Could you check a few things on this model? Use its own coordinates, in mm. A direction names the side the tool comes from. Coordinates: 2 decimals unless noted, no trailing zeros. Loops run counter-clockwise (first coordinate to the right, second up) from the corner with the lowest first, then second, coordinate; pieces in that order, holes last.
from build123d import *

# Parameters (mm, degrees)
BOSS_EXTRUDE1_DEPTH = 5
SKETCH2_W           = 236
SKETCH2_H           = 306
SKETCH2_W_2         = 230
SKETCH2_H_2         = 300
BOSS_EXTRUDE2_DEPTH = 50


with BuildPart() as part:
    # Sketch1 → Boss-Extrude1 (new body)
    with BuildSketch(Plane(origin=(0, 0, 0), x_dir=(1, 0, 0), z_dir=(0, 1, 0))):
        Polygon((-115, 150), (115, 150), (115, 115), (65, 115), (65, 65), (115, 65), (115, -5), (65, -5), (65, -55), (115, -55), (115, -150), (-115, -150), (-115, -55), (-65, -55), (-65, -5), (-115, -5), (-115, 65), (-65, 65), (-65, 115), (-115, 115), align=None)
    extrude(amount=BOSS_EXTRUDE1_DEPTH)

    # Sketch2 → Boss-Extrude2 (add)
    with BuildSketch(Plane(origin=(0, 0, 0), x_dir=(1, 0, 0), z_dir=(0, 1, 0))):
        Rectangle(SKETCH2_W, SKETCH2_H)
        Rectangle(SKETCH2_W_2, SKETCH2_H_2, mode=Mode.SUBTRACT)
    extrude(amount=BOSS_EXTRUDE2_DEPTH)


solid = part.part
(1) I need wall thicknesses on probe 1 along X at (y, z) = (39, 4.5); probe 2 along Z at (x, y) = (35, 33); probe 3 along Y at (x, z) = (-11, -21). Which ranges of each line are inside material? Lowest first, please.
Answers:
probe 1: x = -118 to -115, 115 to 118
probe 2: z = -153 to -150, 150 to 153
probe 3: y = 0 to 5
(2) Imagine slicing it at B-B, the plane y = 32. Write out the boundary of the cut face in (x, z).
Answers:
outline: (-118, -153) - (118, -153) - (118, 153) - (-118, 153) - close; hole (-115, -150) - (115, -150) - (115, 150) - (-115, 150) - close
(3) For pin 1 (12 mm diameter, centred on x = -89, z = -7.5, fed in from +Y), with a flat end and sliding along its axis, tell me the tip position at first contact or that it passes through.
Answers:
pin 1: stops at y = 5
(4) Imagine slicing it at C-C, the plane z = -105. Write out the boundary of the cut face in (x, y), and give its area (3 significant figures).
Answers:
outline: (-118, 0) - (-115, 0) - (-115, 50) - (-118, 50) - close; (-65, 0) - (65, 0) - (65, 5) - (-65, 5) - close; (115, 0) - (118, 0) - (118, 50) - (115, 50) - close
area: 950 mm2
(5) Imagine slicing it at D-D, the plane x = 28.5. Write out the boundary of the cut face in (y, z), and give its area (3 significant figures).
Answers:
outline: (0, -153) - (50, -153) - (50, -150) - (5, -150) - (5, 150) - (50, 150) - (50, 153) - (0, 153) - close
area: 1,800 mm2
(6) We'd pull the mould along Z, two halves only. Please class faces 1 (the face through (115, 25, 2)), 2 (the face through (-2, 27, 150)), 3 (the face through (-2, 0, -2)), 4 (the face through (-2, 25, 153)): +Z half, -Z half, draft (parallel to the pull), parting line (faces both ways), or undercut.
Answers:
face 1: undercut
face 2: undercut
face 3: draft
face 4: +Z half
(7) Imagine slicing it at A-A, the plane x = 74. Write out the boundary of the cut face in (y, z).
Answers:
outline: (0, -153) - (50, -153) - (50, -150) - (5, -150) - (5, -115) - (0, -115) - close; (0, -65) - (5, -65) - (5, 5) - (0, 5) - close; (0, 55) - (5, 55) - (5, 150) - (50, 150) - (50, 153) - (0, 153) - close
(8) Which directions (+Z, -Z, +X, -X, +Y, -Y) give clear straight access to the entire face, cutting with the end or side of a thin tool? Please do faces 5 (the face through (-115, 25, 2)), 6 (the face through (-2, 25, -153)).
Answers:
face 5: +Y
face 6: -Z, +X, -X, +Y, -Y
